Part model, mm, in its own coordinate system. Coordinates: 2 decimals unless noted, no trailing zeros. Loops run counter-clockwise (first coordinate to the right, second up) from the corner with the lowest first, then second, coordinate; pieces in that order, holes last. Notation, with made-up numbers: (11.25, -3.75) - (55.25, -3.75) arc R16 cw to (55.25, 24.25) - close; hole circle Ø6 at (27, -1). An arc over 180 degrees is marked (long way). Answer as CSV lines item,"result".
Autodesk Inventor part; units mm, degrees
ref_plane "YZ Plane" through (0, 0, 0) normal (1, 0, 0) x (0, 1, 0)
ref_plane "XZ Plane" through (0, 0, 0) normal (0, 1, 0) x (-1, 0, 0)
ref_plane "XY Plane" through (0, 0, 0) normal (0, 0, 1) x (1, 0, 0)
sketch "Sketch1" plane through (0, 0, 0) normal (0, 1, 0) x (-1, 0, 0)
  line L0 (-666.6265, 392.3922) -> (-666.6265, -14.0078)
  line L1 (6.4735, -14.0078) -> (6.4735, 392.3922)
  line L2 (-196.7265, 392.3922) -> (-196.7265, 525.7422)
  line L3 (-196.7265, 525.7422) -> (-463.4265, 525.7422)
  line L4 (-463.4265, 525.7422) -> (-463.4265, 392.3922)
  line L5 (6.4735, 392.3922) -> (-196.7265, 392.3922)
  line L6 (-463.4265, 392.3922) -> (-666.6265, 392.3922)
  line L7 (-196.7265, -14.0078) -> (-196.7265, -147.3578)
  line L8 (-196.7265, -147.3578) -> (-463.4265, -147.3578)
  line L9 (-463.4265, -147.3578) -> (-463.4265, -14.0078)
  line L10 (-666.6265, -14.0078) -> (-463.4265, -14.0078)
  line L11 (-196.7265, -14.0078) -> (6.4735, -14.0078)
  point P0 (0, 0)
  dimension "d0" = 673.1
  dimension "d1" = 406.4
  dimension "d73" = 266.7
  dimension "d75" = 203.2
  dimension "d76" = 266.7
extrude "Extrusion1" add sketch "Sketch1" along normal blind 12.7
sketch "Sketch2" plane through (0, 12.7, 0) normal (0, 1, 0) x (1, 0, 0)
  line L0 (666.6265, -392.3922) -> (666.6265, 14.0078)
  line L1 (666.6265, -392.3922) -> (666.6265, -290.7922)
  line L2 (666.6265, -290.7922) -> (666.6265, -189.1922) construction
  line L3 (666.6265, 14.0078) -> (666.6265, -58.7236) construction
  line L4 (666.6265, 14.0078) -> (666.6265, -87.5922) construction
  line L5 (-6.4735, 14.0078) -> (-6.4735, -392.3922) construction
  line L6 (-6.4735, -392.3922) -> (241.1765, -392.3922) construction
  line L7 (-6.4735, -392.3922) -> (666.6265, -392.3922) construction
  line L8 (666.6265, -392.3922) -> (418.9765, -392.3922) construction
  circle A0 centre (653.9265, -290.7922) radius 3.175
  circle A1 centre (653.9265, -87.5922) radius 3.175
  circle A2 centre (241.1765, -379.6922) radius 3.175
  circle A3 centre (418.9765, -379.6922) radius 3.175
  circle A4 centre (418.9765, 1.3078) radius 3.175
  circle A5 centre (241.1765, 1.3078) radius 3.175
  circle A6 centre (6.2265, -87.5922) radius 3.175
  circle A7 centre (6.2265, -290.7922) radius 3.175
  circle A8 centre (6.2265, -239.9922) radius 3.9751
  circle A9 centre (6.2265, -138.3922) radius 3.9751
  circle A10 centre (653.9265, -239.9922) radius 3.9751
  circle A11 centre (653.9265, -138.3922) radius 3.9751
  line L9 (458.3979, 14.0078) -> (460.8865, 14.0078)
  line L10 (460.8865, 14.0078) -> (460.8865, -3.7722)
  line L11 (460.8865, -3.7722) -> (448.1865, -3.7722)
  line L12 (448.1865, -3.7722) -> (448.1865, 7.197)
  line L13 (448.1865, 7.197) -> (460.8865, 7.197)
  line L14 (460.8865, 7.197) -> (460.8865, -3.7722)
  line L15 (666.6265, 14.0078) -> (-6.4735, 14.0078)
  circle A12 centre (330.0765, -513.0422) radius 3.9751
  line L16 (196.7265, -392.3922) -> (196.7265, -525.7422)
  circle A13 centre (330.0765, 134.6578) radius 3.9751
  line L17 (196.7265, 147.3578) -> (196.7265, 14.0078)
  line L18 (196.7265, -525.7422) -> (463.4265, -525.7422)
  line L19 (463.4265, 147.3578) -> (196.7265, 147.3578)
  point P0 (0, 0)
  dimension "d11" = 6.35
  dimension "d12" = 6.35
  dimension "d13" = 12.7
  dimension "d14" = 12.7
  dimension "d15" = 6.35
  dimension "d16" = 12.7
  dimension "d17" = 6.35
  dimension "d18" = 12.7
  dimension "d19" = 6.35
  dimension "d20" = 6.35
  dimension "d23" = 6.35
  dimension "d24" = 6.35
  dimension "d25" = 12.7
  dimension "d26" = 12.7
  dimension "d34" = 7.9502
  dimension "d35" = 7.9502
  dimension "d40" = 50.8
  dimension "d43" = 50.8
  dimension "d44" = 7.9502
  dimension "d45" = 7.9502
  dimension "d46" = 50.8
  dimension "d66" = 205.74
  dimension "d68" = 12.7
  dimension "d70" = 17.78
  dimension "d78" = 7.9502
  dimension "d79" = 133.35
  dimension "d80" = 7.9502
  dimension "d81" = 133.35
  dimension "d82" = 12.7
  dimension "d83" = 12.7
hole "Hole1" at (653.9265, 12.7, 290.7922) at (653.9265, 12.7, 87.5922) at (418.9765, 12.7, -1.3078) at (241.1765, 12.7, -1.3078) at (418.9765, 12.7, 379.6922) at (241.1765, 12.7, 379.6922) at (6.2265, 12.7, 290.7922) at (6.2265, 12.7, 87.5922) at (6.2265, 12.7, 239.9922) at (6.2265, 12.7, 138.3922) at (653.9265, 12.7, 239.9922) at (653.9265, 12.7, 138.3922) at (330.0765, 12.7, 513.0422) at (330.0765, 12.7, -134.6578) direction (0, -1, 0) diameter 7.9502 end through all
sketch "Sketch3" plane through (0, 12.7, 0) normal (0, 1, 0) x (1, 0, 0)
  line L0 (-6.4735, -392.3922) -> (666.6265, -392.3922)
  line L1 (-6.4735, -392.3922) -> (63.1225, -392.3922)
  line L2 (63.1225, -392.3922) -> (63.1225, -366.9922)
  line L3 (63.1225, -366.9922) -> (18.9265, -366.9922)
  line L4 (-6.4735, -366.9922) -> (-6.4735, -392.3922)
  line L5 (-6.4735, -392.3922) -> (18.9265, -392.3922)
  line L6 (18.9265, -366.9922) -> (18.9265, -322.7962)
  line L7 (18.9265, -322.7962) -> (-6.4735, -322.7962)
  line L8 (-6.4735, -322.7962) -> (-6.4735, -392.3922)
  line L9 (666.6265, 14.0078) -> (-6.4735, 14.0078)
  line L10 (-6.4735, 14.0078) -> (63.1225, 14.0078)
  line L11 (63.1225, 14.0078) -> (63.1225, -11.3922)
  line L12 (63.1225, -11.3922) -> (18.9265, -11.3922)
  line L13 (-6.4735, -11.3922) -> (-6.4735, 14.0078)
  line L14 (-6.4735, 14.0078) -> (18.9265, 14.0078)
  line L15 (18.9265, -11.3922) -> (18.9265, -55.5882)
  line L16 (18.9265, -55.5882) -> (-6.4735, -55.5882)
  line L17 (-6.4735, -55.5882) -> (-6.4735, 14.0078)
  line L18 (666.6265, -392.3922) -> (641.2265, -392.3922)
  line L19 (641.2265, -366.9922) -> (641.2265, -322.7962)
  line L20 (641.2265, -322.7962) -> (666.6265, -322.7962)
  line L21 (666.6265, -322.7962) -> (666.6265, -392.3922)
  line L22 (666.6265, -392.3922) -> (597.0305, -392.3922)
  line L23 (597.0305, -392.3922) -> (597.0305, -366.9922)
  line L24 (597.0305, -366.9922) -> (641.2265, -366.9922)
  line L25 (666.6265, -366.9922) -> (666.6265, -392.3922)
  line L26 (666.6265, 14.0078) -> (597.0305, 14.0078)
  line L27 (597.0305, 14.0078) -> (597.0305, -11.3922)
  line L28 (597.0305, -11.3922) -> (641.2265, -11.3922)
  line L29 (666.6265, -11.3922) -> (666.6265, 14.0078)
  line L30 (666.6265, 14.0078) -> (641.2265, 14.0078)
  line L31 (641.2265, -11.3922) -> (641.2265, -55.5882)
  line L32 (641.2265, -55.5882) -> (666.6265, -55.5882)
  line L33 (666.6265, -55.5882) -> (666.6265, 14.0078)
  point P0 (0, 0)
  dimension "d47" = 69.596
  dimension "d48" = 25.4
  dimension "d49" = 25.4
  dimension "d50" = 69.596
  dimension "d51" = 69.596
  dimension "d52" = 25.4
  dimension "d53" = 25.4
  dimension "d54" = 69.596
  dimension "d55" = 25.4
  dimension "d56" = 69.596
  dimension "d57" = 69.596
  dimension "d58" = 25.4
  dimension "d59" = 69.596
  dimension "d60" = 25.4
  dimension "d61" = 25.4
  dimension "d62" = 69.596
extrude "Extrusion2" cut sketch "Sketch3" against normal blind 25.4
sketch "Sketch4" plane through (0, 12.7, 0) normal (0, 1, 0) x (1, 0, 0)
  line L0 (-6.4735, -55.5882) -> (-6.4735, -322.7962) construction
  line L1 (666.6265, -322.7962) -> (666.6265, -55.5882) construction
  point P0 (0, 0)
properties part number "Polyc_for_swerve" material "Polycarbonate, Clear"
Q1. Saw through at B-B (z = -60.5). Give the cut face in (x, y).
Results:
outline,"(196.73, 0) - (463.43, 0) - (463.43, 12.7) - (196.73, 12.7) - close"
Q2. Saw through at C-C (x = 622). Give the cut face in (y, z).
Results:
outline,"(0, 11.39) - (12.7, 11.39) - (12.7, 366.99) - (0, 366.99) - close"
Q3. Flat gauge pins, fed straight in: pin 1 (6.5 mm diameter, centred on x = 118, y = 9, fed in from -Z); pin 2 (2 mm diameter, centred on y = 2, z = 359, fed in from +X); pin 3 (4 mm diameter, centred on x = 30, y = 8.5, fed in from +Z). Where does each tip first touch, or does it go through?
Results:
pin 1,"stops at z = -14.01"
pin 2,"stops at x = 641.23"
pin 3,"stops at z = 366.99"
Q4. Saw through at A-A (y = 6.5). Count the separate pieces of the cut face and the enclosed holes in it, then the cut area to 3 significant figures.
Results:
separate pieces,"1"
enclosed holes,"14"
area,"332,000 mm^2"
Q5. Wall check: L1, parallel to X at y = 7, z = 237.5; L2, parallel to X at y = 3.5, z = 357.5; L3, parallel to Z at x = 506.5, y = 0.75. Give the ranges that are in metal, low to high.
Results:
L1,"x = -6.47 to 3.13, 9.32 to 650.83, 657.02 to 666.63"
L2,"x = 18.93 to 641.23"
L3,"z = -14.01 to 392.39"
